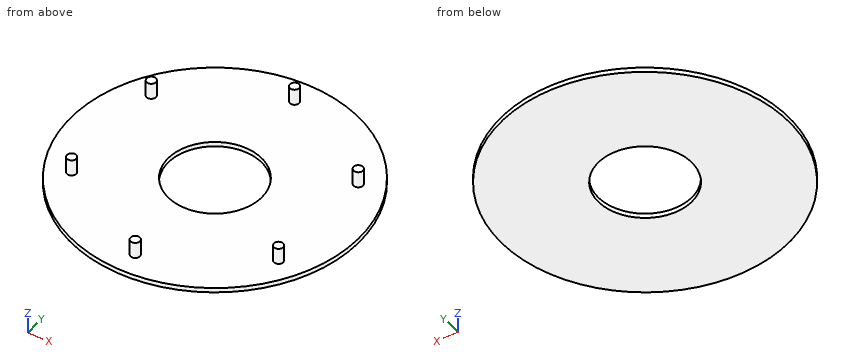
```python
from build123d import *

# Parameters (mm, degrees)
SKETCH1_R           = 61.5
BOSS_EXTRUDE1_DEPTH = 2
SKETCH2_R           = 2
BOSS_EXTRUDE2_DEPTH = 7
CIRPATTERN1_COUNT   = 6
SKETCH1_3_R         = 20
CUT_EXTRUDE1_DEPTH  = 88.255372327


with BuildPart() as part:
    # Sketch1 → Boss-Extrude1 (new body)
    with BuildSketch(Plane.XY):
        Circle(SKETCH1_R)
    extrude(amount=-BOSS_EXTRUDE1_DEPTH)

    # Sketch2 → Boss-Extrude2 (add)
    with BuildSketch(Plane.XY):
        with Locations((0, 51.338311715)):
            Circle(SKETCH2_R)
    boss_extrude2 = extrude(amount=BOSS_EXTRUDE2_DEPTH)

    # CirPattern1: Boss-Extrude2 ×6 about axis
    cirpattern1_axis = Axis((0, 0, 0), (0, 0, 1))
    for i in range(1, CIRPATTERN1_COUNT):
        add(boss_extrude2.rotate(cirpattern1_axis, i * 360 / CIRPATTERN1_COUNT))

    # Sketch1_3 → Cut-Extrude1 (cut, through all)
    with BuildSketch(Plane.XY):
        Circle(SKETCH1_3_R)
    extrude(amount=-CUT_EXTRUDE1_DEPTH, mode=Mode.SUBTRACT)


solid = part.part
```
Model file for the job. Use its own axes, mm. Give positions to 0.01 mm unless a question says otherwise; leave off trailing zeros. Loops run counter-clockwise (first coordinate to the right, second up) from the corner with the lowest first, then second, coordinate; pieces in that order, holes last. Notation, with made-up numbers: (1, 12) -> (35, 12) arc R28 cw to (35, 32) -> close; hole circle Ø6 at (67, 10). An arc over 180 degrees is marked (long way). Use CSV: the item, a comma, the result in double quotes. Start each with the question number.
1) Flat gauge pins, fed straight in: pin 1 Ø10 at (x, y) = (17.5, 9.5) entering from +Z; pin 2 Ø10 at (x, y) = (-13, 0.5) entering from +Z; pin 3 Ø1 at (y, z) = (3.5, -0.5) entering from -X; pin 4 Ø1 at (x, z) = (37.5, -0.5) entering from -Y. Where does each tip first touch, or does it go through?
2) Slice it at D-D on x = 49.5. Give the cut face in (y, z).
3) Wall check: line 1 (Y direction, x = 0, z = -0.7); line 2 (Z direction, x = 22, y = -54.5); line 3 (Y direction, x = 5.5, z = -0.5). Give the ranges that are in metal, low to high.
4) Slice it at C-C on z = 4. Give the cut face in (x, y), plus the area to 3 significant figures.
5) Slice it at A-A on x = 0. Give the cut face in (y, z).
6) Slice it at B-B on y = 0. Give the cut face in (x, z), plus the area to 3 significant figures.
Computed values:
1,pin 1,"stops at z = 0"
1,pin 2,"passes through"
1,pin 3,"stops at x = -61.43"
1,pin 4,"stops at y = -49.12"
2,outline,"(-36.5, -2) -> (36.5, -2) -> (36.5, 0) -> (-36.5, 0) -> close"
3,line 1,"y = -61.5 to -20, 20 to 61.5"
3,line 2,"z = -2 to 0"
3,line 3,"y = -61.25 to -19.23, 19.23 to 61.25"
4,outline,"circle Ø4 at (-44.46, -25.67); circle Ø4 at (-44.46, 25.67); circle Ø4 at (0, -51.34); circle Ø4 at (0, 51.34); circle Ø4 at (44.46, -25.67); circle Ø4 at (44.46, 25.67)"
4,area,"75.4 mm^2"
5,outline,"(-61.5, -2) -> (-20, -2) -> (-20, 0) -> (-49.34, 0) -> (-49.34, 7) -> (-53.34, 7) -> (-53.34, 0) -> (-61.5, 0) -> close; (20, -2) -> (61.5, -2) -> (61.5, 0) -> (53.34, 0) -> (53.34, 7) -> (49.34, 7) -> (49.34, 0) -> (20, 0) -> close"
6,outline,"(-61.5, -2) -> (-20, -2) -> (-20, 0) -> (-61.5, 0) -> close; (20, -2) -> (61.5, -2) -> (61.5, 0) -> (20, 0) -> close"
6,area,"166 mm^2"
